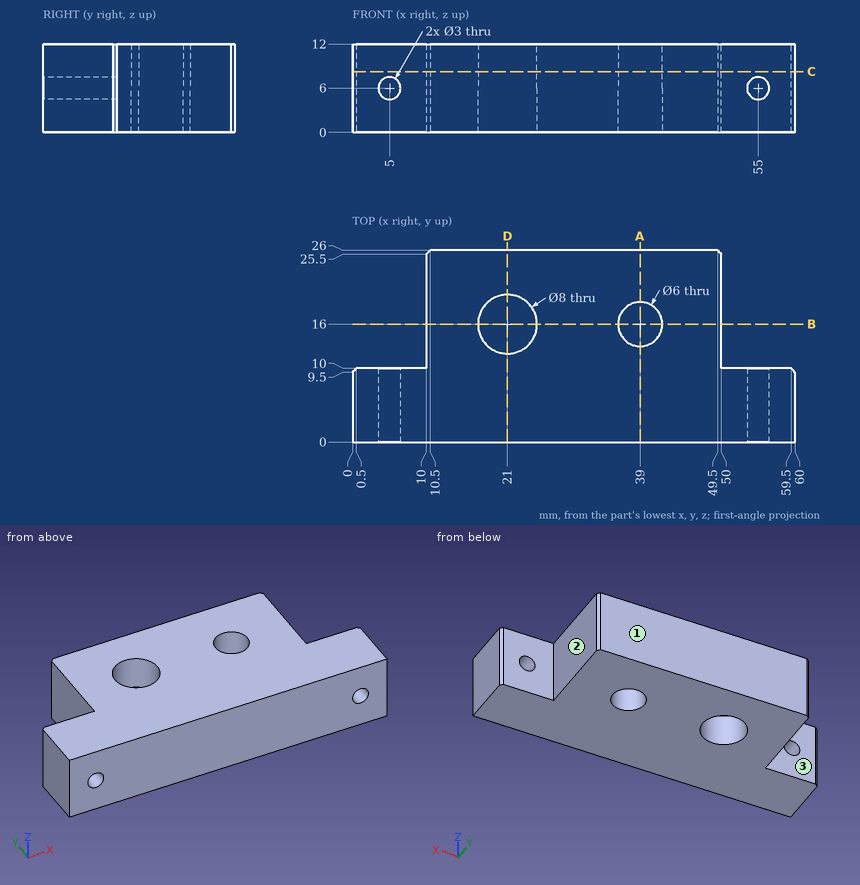
Verification items for this drawing (mm, ordinates from the low corner). A direction names the side the tool comes from. Coordinates: 2 decimals unless noted, no trailing zeros. Write each loop counter-clockwise with the first axis right and the second up, starting at its lowest first coordinate (ties: lowest second). Pieces come first, ordered by that corner, then holes. Notation, with made-up numbers: M 76,34.25 L 96,34.25 A10 ccw 96,48.25 Z; hole C -16,57.5 d8. An arc over 180 degrees is marked long. Answer as CSV lines item,"result".
Q1. Cross-section at A-A (x = 39). Record the boundary of the cut face in (y, z), then the cut area to 3 significant figures.
Check result:
outline,"M 0,0 L 13,0 L 13,12 L 0,12 Z; M 19,0 L 26,0 L 26,12 L 19,12 Z"
area,"240 mm^2"
Q2. Cross-section at D-D (x = 21). Record the boundary of the cut face in (y, z).
Check result:
outline,"M 0,0 L 12,0 L 12,12 L 0,12 Z; M 20,0 L 26,0 L 26,12 L 20,12 Z"
Q3. Cross-section at B-B (y = 16). Record the boundary of the cut face in (x, z), then the cut area to 3 significant figures.
Check result:
outline,"M 10,0 L 17,0 L 17,12 L 10,12 Z; M 25,0 L 36,0 L 36,12 L 25,12 Z; M 42,0 L 50,0 L 50,12 L 42,12 Z"
area,"312 mm^2"
Q4. Cross-section at C-C (z = 8.25). Record the boundary of the cut face in (x, y), then the cut area to 3 significant figures.
Check result:
outline,"M 0,0 L 60,0 L 60,9.5 L 59.5,10 L 50,10 L 50,25.5 L 49.5,26 L 10.5,26 L 10,25.5 L 10,10 L 0.5,10 L 0,9.5 Z; hole C 21,16 d8; hole C 39,16 d6"
area,"1,160 mm^2"
Q5. Go/stop test with flat-tipped pins: pin 1 (5.5 mm diameter, centred on x = 39, y = 16, fed in from -Z); pin 2 (5 mm diameter, centred on x = 5, z = 6, fed in from +Y); pin 3 (1.5 mm diameter, centred on y = 22.5, z = 9.5, fed in from +X). Record where each tip stops, or that it passes through.
Check result:
pin 1,"through"
pin 2,"y = 10"
pin 3,"x = 50"
Q6. Set-up check for the marked faces 1, 2 and 3: record each of +Z, -Z, +X, -X, +Y, -Y from which the full face is reachable in a straight line by a thin tool's end or side.
Check result:
face 1,"+Z, -Z, +X, -X, +Y"
face 2,"+Z, -Z, +X, +Y"
face 3,"+Z, -Z, -X, +Y"
Q7. Material ranges on probe 1 along Y at (x, z) = (21, 1.6); probe 2 along Z at (x, y) = (55, 7.5); probe 3 along X at (y, z) = (17.75, 4), recorded low to high. Write a range as from..to.
Check result:
probe 1,"0..12, 20..26"
probe 2,"0..4.5, 7.5..12"
probe 3,"10..17.4, 24.6..36.56, 41.44..50"
